Read the model definition and answer for the solid it produces. Units are mm, in the model's axes. Face numbers are marked on the shaded views. A direction names the side the tool comes from. Give positions to 0.01 mm unless a question says otherwise; leave off trailing zeros. Loops run counter-clockwise (first coordinate to the right, second up) from the corner with the lowest first, then second, coordinate; pieces in that order, holes last. Notation, with made-up numbers: (71.5, -31) - (124.5, -31) arc R31 ccw to (124.5, -4) - close; hole circle Ø3 at (-33, -35.5). An arc over 180 degrees is marked (long way). Write item = value, one per line.
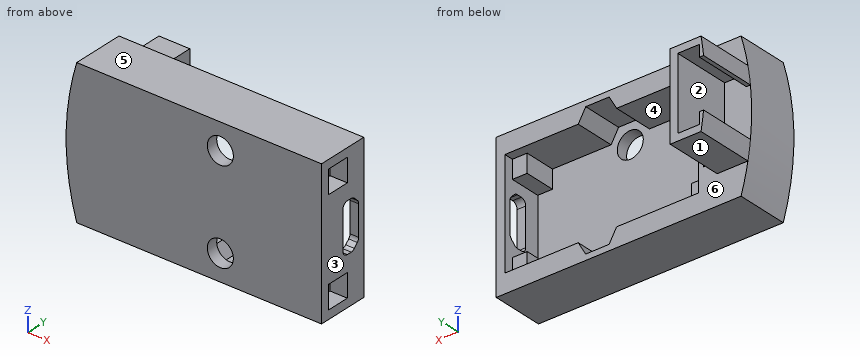
```python
from build123d import *

# Parameters (mm, degrees)
BOSS_EXTRUDE1_DEPTH  = 9
SKETCH17_W           = 33.5
SKETCH17_H           = 18.5
CUT_EXTRUDE8_DEPTH   = 7
SKETCH18_W           = 2.55
SKETCH18_H           = 3.15
BOSS_EXTRUDE2_DEPTH  = 5.4
CUT_EXTRUDE13_REACH  = 49.509
CUT_EXTRUDE15_REACH  = 30.68
SKETCH27_R           = 2.25
CUT_EXTRUDE14_DEPTH  = 7
SKETCH28_W           = 2.4
SKETCH28_H           = 11
CUT_EXTRUDE16_DEPTH  = 5
SKETCH29_W           = 4
SKETCH29_H           = 4
CUT_EXTRUDE17_DEPTH  = 3
BOSS_EXTRUDE4_DEPTH  = 10
SKETCH33_OUTSIDE_W   = 57.507
SKETCH33_OUTSIDE_H   = 43.336
SKETCH33_OUTSIDE_W_2 = 61.074574046
SKETCH33_OUTSIDE_H_2 = 25
CUT_EXTRUDE24_DEPTH  = 34.683188999


with BuildPart() as part:
    # Sketch1 → Boss-Extrude1 (new body)
    with BuildSketch(Plane(origin=(0, 0, 0), x_dir=(1, 0, 0), z_dir=(0, 1, 0))):
        with BuildLine():
            Line((-20.75, 15), (20.75, 15))
            Line((20.75, 15), (20.75, -15))
            Line((20.75, -15), (-20.75, -15))
            ThreePointArc((-20.75, -15), (-23.421298451, 0), (-20.75, 15))
        make_face()
    extrude(amount=BOSS_EXTRUDE1_DEPTH)

    # Sketch17 → Cut-Extrude8 (cut)
    with BuildSketch(Plane(origin=(0, 9, 0), x_dir=(1, 0, 0), z_dir=(0, 1, 0))):
        with Locations((2.5, 0)):
            Rectangle(SKETCH17_W, SKETCH17_H)
    extrude(amount=-CUT_EXTRUDE8_DEPTH, mode=Mode.SUBTRACT)

    # Sketch18 → Boss-Extrude2 (add)
    with BuildSketch(Plane(origin=(0, 2, 0), x_dir=(1, 0, 0), z_dir=(0, 1, 0))):
        with Locations((-12.975, 7.675)):
            Rectangle(SKETCH18_W, SKETCH18_H)
        with Locations((-12.975, -7.675)):
            Rectangle(SKETCH18_W, SKETCH18_H)
        with Locations((17.975, 7.675)):
            Rectangle(SKETCH18_W, SKETCH18_H)
        with Locations((17.975, -7.675)):
            Rectangle(SKETCH18_W, SKETCH18_H)
    extrude(amount=BOSS_EXTRUDE2_DEPTH)

    # Sketch25 → Cut-Extrude13 (cut, up to next)
    with BuildSketch(Plane(origin=(20.75, 0, 0), x_dir=(0, 0, -1), z_dir=(1, 0, 0)), mode=Mode.PRIVATE) as cut_extrude13_sk1:
        with BuildLine():
            Line((3.921751442, 6.999799178), (3.28890873, 7.63264189))
            ThreePointArc((3.28890873, 7.63264189), (2.980706548, 7.838576004), (2.617157288, 7.910890448))
            Line((2.617157288, 7.910890448), (-2.617157288, 7.910890448))
            ThreePointArc((-2.617157288, 7.910890448), (-2.980706548, 7.838576004), (-3.28890873, 7.63264189))
            Line((-3.28890873, 7.63264189), (-3.921751442, 6.999799178))
            ThreePointArc((-3.921751442, 6.999799178), (-4.127534378, 6.691961757), (-4.199999672, 6.328837431))
            Line((-4.199999672, 6.328837431), (-4.2, 5.510890448))
            ThreePointArc((-4.2, 5.510890448), (-3.921751442, 4.839139006), (-3.25, 4.560890448))
            Line((-3.25, 4.560890448), (3.25, 4.560890448))
            ThreePointArc((3.25, 4.560890448), (3.921751442, 4.839139006), (4.2, 5.510890448))
            Line((4.2, 5.510890448), (4.2, 6.329548061))
            Line((4.2, 6.329548061), (4.199995261, 6.331048392))
            ThreePointArc((4.199995261, 6.331048392), (4.12711031, 6.692982667), (3.921751442, 6.999799178))
        make_face()
    cut_extrude13_tool1 = extrude(cut_extrude13_sk1.sketch, amount=-CUT_EXTRUDE13_REACH, mode=Mode.PRIVATE) & part.part
    add(cut_extrude13_tool1.solids().sort_by_distance((20.75, 6.185522, 0))[0], mode=Mode.SUBTRACT)

    # Sketch27 → Cut-Extrude15 (cut, up to next)
    with BuildSketch(Plane(origin=(0, 2, 0), x_dir=(1, 0, 0), z_dir=(0, 1, 0)), mode=Mode.PRIVATE) as cut_extrude15_sk1:
        with Locations(Location((3.25, -8, 0), (0, 0, 326.251011404))):
            Circle(SKETCH27_R)
    cut_extrude15_tool1 = extrude(cut_extrude15_sk1.sketch, amount=-CUT_EXTRUDE15_REACH, mode=Mode.PRIVATE) & part.part
    # Sketch27 → Cut-Extrude15 (cut, up to next)
    with BuildSketch(Plane(origin=(0, 2, 0), x_dir=(1, 0, 0), z_dir=(0, 1, 0)), mode=Mode.PRIVATE) as cut_extrude15_sk2:
        with Locations(Location((3.25, 8, 0), (0, 0, 33.748988596))):
            Circle(SKETCH27_R)
    cut_extrude15_tool2 = extrude(cut_extrude15_sk2.sketch, amount=-CUT_EXTRUDE15_REACH, mode=Mode.PRIVATE) & part.part
    add(cut_extrude15_tool1.solids().sort_by_distance((3.25, 2, 8))[0], mode=Mode.SUBTRACT)
    add(cut_extrude15_tool2.solids().sort_by_distance((3.25, 2, -8))[0], mode=Mode.SUBTRACT)

    # Sketch26 → Cut-Extrude14 (cut)
    with BuildSketch(Plane(origin=(0, 9, 0), x_dir=(1, 0, 0), z_dir=(0, 1, 0))):
        Polygon((5.270725942, -4.5), (1.229274058, -4.5), (-0.791451884, -8), (1.229274058, -11.5), (5.270725942, -11.5), (7.291451884, -8), align=None)
        Polygon((7.291451884, 8), (5.270725942, 4.5), (1.229274058, 4.5), (-0.791451884, 8), (1.229274058, 11.5), (5.270725942, 11.5), align=None)
    extrude(amount=-CUT_EXTRUDE14_DEPTH, mode=Mode.SUBTRACT)

    # Sketch28 → Cut-Extrude16 (cut)
    with BuildSketch(Plane(origin=(0, 9, 0), x_dir=(1, 0, 0), z_dir=(0, 1, 0))):
        with Locations((-16.25, 0)):
            Rectangle(SKETCH28_W, SKETCH28_H)
    extrude(amount=-CUT_EXTRUDE16_DEPTH, mode=Mode.SUBTRACT)

    # Sketch29 → Cut-Extrude17 (cut)
    with BuildSketch(Plane(origin=(20.75, 0, 0), x_dir=(0, 0, -1), z_dir=(1, 0, 0))):
        with Locations((-9, 3.5)):
            Rectangle(SKETCH29_W, SKETCH29_H)
        with Locations((9, 3.5)):
            Rectangle(SKETCH29_W, SKETCH29_H)
    extrude(amount=-CUT_EXTRUDE17_DEPTH, mode=Mode.SUBTRACT)

    # Sketch32 → Boss-Extrude4 (add)
    with BuildSketch(Plane(origin=(0, 9, 0), x_dir=(1, 0, 0), z_dir=(0, 1, 0))):
        with BuildLine():
            Line((-22.005035217, 6.25), (-18.755035217, 6.25))
            Line((-18.755035217, 6.25), (-18.755035217, -6.25))
            Line((-18.755035217, -6.25), (-22.505035217, -6.25))
            Line((-22.505035217, -6.25), (-22.505035217, -4.25))
            Line((-22.505035217, -4.25), (-23.212945043, -4.25))
            ThreePointArc((-23.212945043, -4.25), (-23.025133018, -5.854043824), (-22.777840007, -7.45))
            Line((-22.777840007, -7.45), (-17.45, -7.45))
            Line((-17.45, -7.45), (-17.45, -5.5))
            Line((-17.45, -5.5), (-17.45, 5.5))
            Line((-17.45, 5.5), (-17.45, 7.45))
            Line((-17.45, 7.45), (-22.777840007, 7.45))
            ThreePointArc((-22.777840007, 7.45), (-23.025133018, 5.854043824), (-23.212945043, 4.25))
            Line((-23.212945043, 4.25), (-22.505035217, 4.25))
            Line((-22.505035217, 4.25), (-22.505035217, 6.25))
            Line((-22.505035217, 6.25), (-22.005035217, 6.25))
        make_face()
    extrude(amount=BOSS_EXTRUDE4_DEPTH)

    # Sketch33 outside → Cut-Extrude24 (cut, through all)
    with BuildSketch(Plane(origin=(0, 0, 0), x_dir=(1, 0, 0), z_dir=(0, 1, 0))):
        with Locations((-1.3355, 0)):
            Rectangle(SKETCH33_OUTSIDE_W, SKETCH33_OUTSIDE_H)
        Rectangle(SKETCH33_OUTSIDE_W_2, SKETCH33_OUTSIDE_H_2, mode=Mode.SUBTRACT)
    extrude(amount=CUT_EXTRUDE24_DEPTH, mode=Mode.SUBTRACT)


solid = part.part
```
1) Find the intervals of material crossed by probe 1 along Z at (x, y) = (3.25, 1.65); probe 2 along Z at (x, y) = (-9.5, 5); probe 3 along X at (y, z) = (10.25, -1), in increasing order.
Output:
probe_1 = -12.5 to -10.25, -5.75 to 5.75, 10.25 to 12.5
probe_2 = -12.5 to -9.25, 9.25 to 12.5
probe_3 = -18.76 to -17.45
2) A cutting plane is placed at C-C on x = -2.5. Determine the outline of the cut face in (y, z), then the cut area to 3 significant figures.
Output:
outline = (0, -12.5) - (9, -12.5) - (9, -9.25) - (2, -9.25) - (2, 9.25) - (9, 9.25) - (9, 12.5) - (0, 12.5) - close
area = 95.5 mm²
3) A tool of negligible diameter and unlimited length cuts with its end or side. For the marked faces 1, 2 and 3, from which of +Z, -Z, +X, -X, +Y, -Y can it reach the whole face along a straight path? Write none if from no direction.
Output:
face_1 = -Z, +X, -X, +Y
face_2 = +Y
face_3 = +Z, -Z, +X, +Y, -Y
4) A cutting plane is placed at D-D on y = 17.5. Determine the outline of the cut face in (x, z).
Output:
outline = (-23.21, -4.25) arc R43.45 ccw to (-22.78, -7.45) - (-17.45, -7.45) - (-17.45, 7.45) - (-22.78, 7.45) arc R43.45 ccw to (-23.21, 4.25) - (-22.51, 4.25) - (-22.51, 6.25) - (-18.76, 6.25) - (-18.76, -6.25) - (-22.51, -6.25) - (-22.51, -4.25) - close
5) Each of these flat-tipped pins is pushed along its axis until it touches: P1, Ø2.5, axis at y = 6, z = 7.5, coming from the -X side; P2, Ø0.8, axis at x = 20, z = 1, coming from the +Y side; P3, Ø2, axis at y = 3, z = 9.5, coming from the +X side. Where does it stop, or does it pass through?
Output:
P1 = -22.97
P2 = 9
P3 = 17.75
6) A cutting plane is placed at A-A on x = 3.25. Determine the outline of the cut face in (y, z).
Output:
outline = (0, -12.5) - (9, -12.5) - (9, -11.5) - (2, -11.5) - (2, -10.25) - (0, -10.25) - close; (0, -5.75) - (2, -5.75) - (2, 5.75) - (0, 5.75) - close; (0, 10.25) - (2, 10.25) - (2, 11.5) - (9, 11.5) - (9, 12.5) - (0, 12.5) - close
7) A cutting plane is placed at B-B on z = 1. Determine the outline of the cut face in (x, y).
Output:
outline = (-23.41, 0) - (20.75, 0) - (20.75, 4.56) - (19.25, 4.56) - (19.25, 2) - (-14.25, 2) - (-14.25, 9) - (-15.05, 9) - (-15.05, 4) - (-17.45, 4) - (-17.45, 19) - (-18.76, 19) - (-18.76, 9) - (-23.41, 9) - close; (19.25, 7.91) - (20.75, 7.91) - (20.75, 9) - (19.25, 9) - close
8) The mould has two halves that part along Z. Classify the marked faces 4, 5 and 6: pulls with the +Z half, pulls with the -Z half, needs draft (parallel to the pull), parting line crosses it, or undercut.
Output:
face_4 = undercut
face_5 = pulls with the +Z half
face_6 = needs draft
